Input: dimensioned drawing with shaded views. Units: mm. Origin: part minimum x, y, z. A direction names the side the tool comes from. Round coordinates to 2 decimals unless told otherwise and drop trailing zeros. Loops run counter-clockwise (first coordinate to the right, second up) from the corner with the lowest first, then second, coordinate; pieces in that order, holes last. Notation, with made-up numbers: (-32, 51) -> (13, 51) arc R11 ccw to (13, 55) -> close; hole circle Ø6 at (87, -25). An arc over 180 degrees is marked (long way). Answer as a JSON object with one key per item and string values.
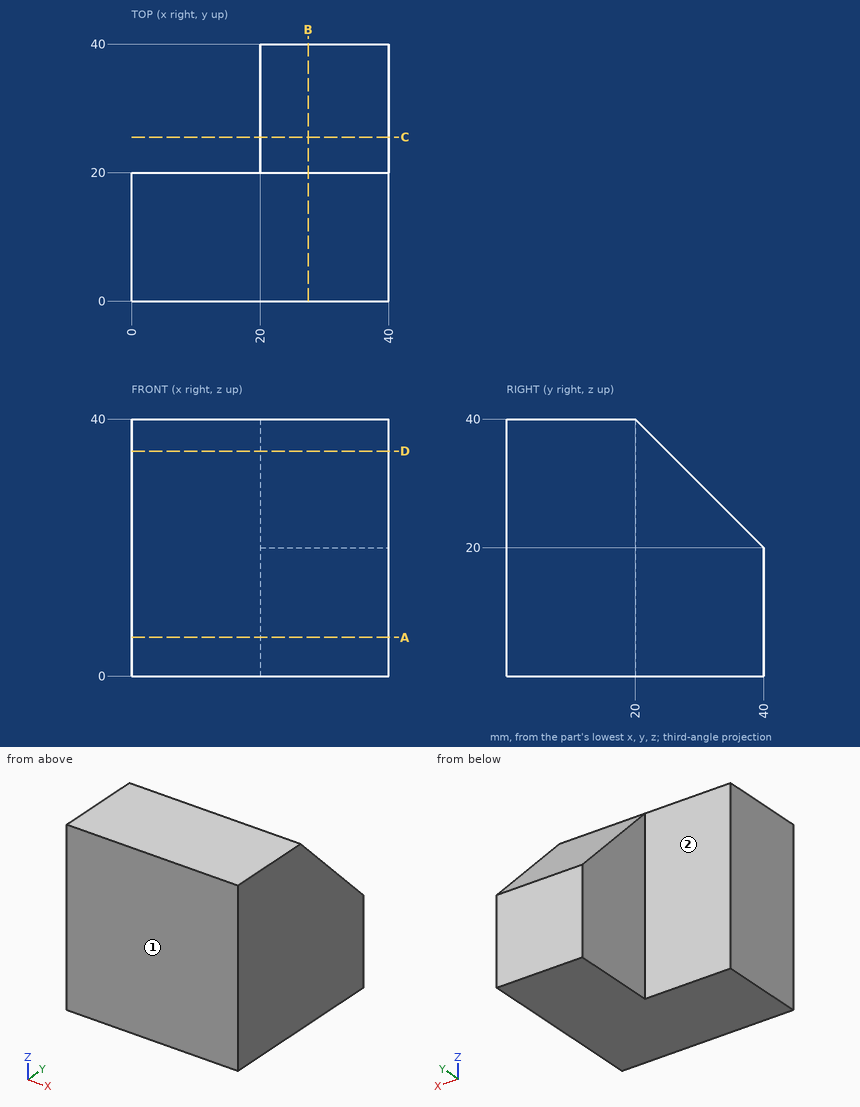
1) Ray query, probe 1 along Y at (x, z) = (14, 4.5); probe 2 along X at (y, z) = (37.5, 12); probe 3 along Y at (x, z) = (25, 25.5). Return the intervals inside material, ascending.
Output:
{"probe 1": "y = 0 to 20", "probe 2": "x = 20 to 40", "probe 3": "y = 0 to 34.5"}
2) Contact query for flat-ended pins moving along their axis: P1, Ø8, axis at x = 17, y = 36, coming from the -Z side; P2, Ø10, axis at x = 13, z = 14, coming from the +Y side; P3, Ø10, axis at y = 26.5, z = 16, coming from the -X side. Output: stop coordinate, or through.
Output:
{"P1": "stops at z = 0", "P2": "stops at y = 20", "P3": "stops at x = 20"}
3) Section B-B, the plane x = 27.5. Output: boundary loops of the cut face in (y, z).
Output:
{"outline": "(0, 0) -> (40, 0) -> (40, 20) -> (20, 40) -> (0, 40) -> close"}
4) Section C-C, the plane y = 25.5. Output: boundary loops of the cut face in (x, z), plus the area to 3 significant figures.
Output:
{"outline": "(20, 0) -> (40, 0) -> (40, 34.5) -> (20, 34.5) -> close", "area": "690 mm^2"}
5) Section D-D, the plane z = 35. Output: boundary loops of the cut face in (x, y), plus the area to 3 significant figures.
Output:
{"outline": "(0, 0) -> (40, 0) -> (40, 25) -> (20, 25) -> (20, 20) -> (0, 20) -> close", "area": "900 mm^2"}
6) Reachability of the marked faces 1 and 2 from +Z, -Z, +X, -X, +Y, -Y: full face, straight path, thin tool, end or side. Return the list, or none.
Output:
{"face 1": "+Z, -Z, +X, -X, -Y", "face 2": "+Z, -Z, -X, +Y"}
7) Section A-A, the plane z = 6. Output: boundary loops of the cut face in (x, y), plus the area to 3 significant figures.
Output:
{"outline": "(0, 0) -> (40, 0) -> (40, 40) -> (20, 40) -> (20, 20) -> (0, 20) -> close", "area": "1,200 mm^2"}
